Geometry: final body of the model. Coordinates: model frame, mm. A direction names the side the tool comes from. Round coordinates to 2 decimals unless told otherwise and drop trailing zeros. Loops run counter-clockwise (first coordinate to the right, second up) from the corner with the lowest first, then second, coordinate; pieces in that order, holes last. Notation, with made-up numbers: M 50.5,15 L 69.5,15 A19 cw 69.5,51 Z; hole C 15,51 d9. An arc over 180 degrees is marked long. Return JSON: item names as keys, results as strings.
from build123d import *

# Parameters (mm, degrees)
F0_R     = 15.875
F1_DEPTH = 31.75
F2_R     = 6.35
F3_DEPTH = 44.45
F4_R     = 4.445
F5_DEPTH = 69.85


with BuildPart() as f1:
    # F0 (on Top) → F1 (new body)
    with BuildSketch(Plane.XY):
        Circle(F0_R)
    extrude(amount=F1_DEPTH)

    # F2 (on face) → F3 (join)
    with BuildSketch(Plane(origin=(0, 0, 0), x_dir=(1, 0, 0), z_dir=(0, 0, -1))):
        Circle(F2_R)
    extrude(amount=F3_DEPTH)

    # F4 (on Front) → F5 (join, symmetric)
    with BuildSketch(Plane.XZ):
        with Locations((0, 15.875)):
            Circle(F4_R)
    extrude(amount=F5_DEPTH, both=True)

    # F6 (on Right) → F7 (revolve)
    with BuildSketch(Plane.YZ):
        with BuildLine():
            Line((69.85, 20.32), (69.85, 15.875))
            Line((69.85, 15.875), (89.146059, 15.875))
            ThreePointArc((89.146059, 15.875), (81.266765, 25.775706), (69.85, 20.32))
        make_face()
        with BuildLine():
            ThreePointArc((-69.85, 20.32), (-81.266765, 25.775706), (-89.146059, 15.875))
            Line((-89.146059, 15.875), (-69.85, 15.875))
            Line((-69.85, 15.875), (-69.85, 20.32))
        make_face()
    revolve(axis=Axis((0, 79.49803, 15.875), (0, 1, 0)))


solid = f1.part
Q1. Section query A-A (y = 0). Output: boundary loops of the cut face in (x, z) (3 decimals), plus the area to 3 significant figures.
Determined:
{"outline": "M -15.875,0 L -6.35,0 L -6.35,-44.45 L 6.35,-44.45 L 6.35,0 L 15.875,0 L 15.875,31.75 L -15.875,31.75 Z", "area": "1,570 mm^2"}
Q2. Material intervals for L1, parallel to Y at x = 8.5, z = 18.5; L2, parallel to Z at x = -0.5, y = -65.5; L3, parallel to Y at x = 4, z = 10, sorted ascending.
Determined:
{"L1": "y = -83.89 to -74.08, -13.41 to 13.41, 74.08 to 83.89", "L2": "z = 11.46 to 20.29", "L3": "y = -86.25 to -71.73, -15.36 to 15.36, 71.73 to 86.25"}
Q3. Pin query (flat end, axial travel): pin 1 (2 mm diameter, centred on x = -6.5, z = -26.5, fed in from -Y); pin 2 (1 mm diameter, centred on x = -5, z = -19, fed in from +Y); pin 3 (2 mm diameter, centred on y = 4.5, z = -7.5, fed in from -X); pin 4 (10 mm diameter, centred on x = 12.5, z = -21, fed in from -Y). Return the tip coordinate at first contact, or that it passes through.
Determined:
{"pin 1": "stops at y = -3.17", "pin 2": "stops at y = 4.48", "pin 3": "stops at x = -5.3", "pin 4": "passes through"}
Q4. Reachability of faces 1 (the cylindrical face through (-0.58, 42.15, 20.28)), 2 (the flat face through (0, 0, 31.75)), 3 (the flat face through (7, 0, 0)) from +Z, -Z, +X, -X, +Y, -Y: full face, straight path, thin tool, end or side. Return the list, or none.
Determined:
{"face 1": "none", "face 2": "+Z, +X, -X, +Y, -Y", "face 3": "-Z"}
Q5. Section query D-D (x = 8). Output: boundary loops of the cut face in (y, z) (3 decimals).
Determined:
{"outline": "C -78.986,15.875 d12.526; M -13.712,0 L 13.712,0 L 13.712,31.75 L -13.712,31.75 Z; C 78.986,15.875 d12.526"}
Q6. Section query C-C (z = 17.5). Output: boundary loops of the cut face in (x, y) (3 decimals).
Determined:
{"outline": "M -4.137,-69.85 A10.029 ccw long 4.137,-69.85 L 4.137,-15.326 A15.875 ccw 4.137,15.326 L 4.137,69.85 A10.029 ccw long -4.137,69.85 L -4.137,15.326 A15.875 ccw -4.137,-15.326 Z"}
Q7. Section query B-B (x = 0). Output: boundary loops of the cut face in (y, z) (3 decimals).
Determined:
{"outline": "M -69.85,11.43 L -15.875,11.43 L -15.875,0 L -6.35,0 L -6.35,-44.45 L 6.35,-44.45 L 6.35,0 L 15.875,0 L 15.875,11.43 L 69.85,11.43 A10.16 ccw long 69.85,20.32 L 15.875,20.32 L 15.875,31.75 L -15.875,31.75 L -15.875,20.32 L -69.85,20.32 A10.16 ccw long Z"}
Q8. Pull-direction query (Y, two-part tool) for faces 4 (the flat face through (0, 0, -44.45)), 5 (the cylindrical face through (-1.38, 6.2, -21.91)), 6 (the cylindrical face through (-0.58, -42.92, 20.28)); classes: pulls with the +Y half, pulls with the -Y half, needs draft (parallel to the pull), parting line crosses it, or undercut.
Determined:
{"face 4": "needs draft", "face 5": "parting line crosses it", "face 6": "undercut"}
